Build history of the part. All positions in model axes, mm. Give positions to 0.01 mm unless a question says otherwise; leave off trailing zeros. Loops run counter-clockwise (first coordinate to the right, second up) from the corner with the lowest first, then second, coordinate; pieces in that order, holes last. Notation, with made-up numbers: M 34.25,-0.5 L 43.25,-0.5 A30 cw 43.25,21.5 Z; hole C -33.75,-17.75 d9. An arc over 180 degrees is marked long. Answer as a JSON object with one key per item and string values. Group by question number.
1. Slice it at D-D (z = 37.5). List the corners of the cut face in (x, y).
2. Slice it at A-A (x = -34). List the corners of the cut face in (y, z), then the cut area to 3 significant figures.
3. Slice it at B-B (z = -84.5). List the corners of the cut face in (x, y), then the cut area to 3 significant figures.
4. Drill centre lines: line 1 along X through (y, z) = (2.2, -101); line 2 along X through (y, z) = (2.65, 64); line 3 along X through (y, z) = (1.05, 28). Where is each one in solid material? Low to high. Write a range as [from, to].
5. Slice it at C-C (y = 1.65). Give the number of separate pieces and of enclosed holes in the cut face, then the cut area to 3 significant figures.
from build123d import *

# Parameters (mm, degrees)
SKETCH1_W            = 100
SKETCH1_H            = 210
BOSS_EXTRUDE1_DEPTH  = 3
CUT_EXTRUDE1_REACH   = 118.336
SKETCH3_R            = 1.5
SKETCH3_W            = 2
SKETCH3_H            = 100
LPATTERN1_COUNT      = 2
LPATTERN1_PITCH      = 22.5
CUT_EXTRUDE2_REACH   = 118.336
SKETCH4_W            = 20
SKETCH4_H            = 10
LPATTERN2_COUNT      = 2
LPATTERN2_PITCH      = 22.5
LPATTERN2_COUNT_DIR2 = 2
LPATTERN2_PITCH_DIR2 = 22.5
CUT_EXTRUDE3_REACH   = 118.336
SKETCH5_R            = 1.5
CUT_EXTRUDE4_REACH   = 118.336
SKETCH6_W            = 20
SKETCH6_H            = 10
LPATTERN3_COUNT      = 5
LPATTERN3_PITCH      = 15
CUT_EXTRUDE5_REACH   = 118.336
SKETCH7_R            = 1.5
CUT_EXTRUDE6_REACH   = 118.336
SKETCH8_R            = 1.5


with BuildPart() as part:
    # Sketch1 → Boss-Extrude1 (new body)
    with BuildSketch(Plane(origin=(0, 0, 0), x_dir=(1, 0, 0), z_dir=(0, 1, 0))):
        Rectangle(SKETCH1_W, SKETCH1_H)
    extrude(amount=BOSS_EXTRUDE1_DEPTH)

    # Sketch3 → Cut-Extrude1 (cut, up to next)
    with BuildSketch(Plane(origin=(0, 3, 0), x_dir=(1, 0, 0), z_dir=(0, 1, 0)), mode=Mode.PRIVATE) as cut_extrude1_sk1:
        with Locations(Location((0, -85, 0), (0, 0, 270))):
            Circle(SKETCH3_R)
    cut_extrude1_tool1 = extrude(cut_extrude1_sk1.sketch, amount=-CUT_EXTRUDE1_REACH, mode=Mode.PRIVATE) & part.part
    # Sketch3 → Cut-Extrude1 (cut, up to next)
    with BuildSketch(Plane(origin=(0, 3, 0), x_dir=(1, 0, 0), z_dir=(0, 1, 0)), mode=Mode.PRIVATE) as cut_extrude1_sk2:
        with Locations(Location((0, 35, 0), (0, 0, 270))):
            Circle(SKETCH3_R)
    cut_extrude1_tool2 = extrude(cut_extrude1_sk2.sketch, amount=-CUT_EXTRUDE1_REACH, mode=Mode.PRIVATE) & part.part
    # Sketch3 → Cut-Extrude1 (cut, up to next)
    with BuildSketch(Plane(origin=(0, 3, 0), x_dir=(1, 0, 0), z_dir=(0, 1, 0)), mode=Mode.PRIVATE) as cut_extrude1_sk3:
        with Locations((0, -25)):
            Rectangle(SKETCH3_W, SKETCH3_H)
    cut_extrude1_tool3 = extrude(cut_extrude1_sk3.sketch, amount=-CUT_EXTRUDE1_REACH, mode=Mode.PRIVATE) & part.part
    cut_extrude1_1 = cut_extrude1_tool1.solids().sort_by_distance((0, 3, 85))[0]
    add(cut_extrude1_1, mode=Mode.SUBTRACT)
    cut_extrude1_2 = cut_extrude1_tool2.solids().sort_by_distance((0, 3, -35))[0]
    add(cut_extrude1_2, mode=Mode.SUBTRACT)
    cut_extrude1_3 = cut_extrude1_tool3.solids().sort_by_distance((0, 3, 25))[0]
    add(cut_extrude1_3, mode=Mode.SUBTRACT)
    cut_extrude1 = cut_extrude1_1 + cut_extrude1_2 + cut_extrude1_3  # Cut-Extrude1 as one shape, for the pattern or mirror that repeats it

    # LPattern1: Cut-Extrude1 ×2
    with Locations(*[(i * LPATTERN1_PITCH, 0, 0) for i in range(1, LPATTERN1_COUNT)]):
        add(cut_extrude1, mode=Mode.SUBTRACT)

    # Sketch4 → Cut-Extrude2 (cut, up to next)
    with BuildSketch(Plane(origin=(0, 3, 0), x_dir=(1, 0, 0), z_dir=(0, 1, 0)), mode=Mode.PRIVATE) as cut_extrude2_sk1:
        with Locations((0, 60)):
            Rectangle(SKETCH4_W, SKETCH4_H)
    cut_extrude2_tool1 = extrude(cut_extrude2_sk1.sketch, amount=-CUT_EXTRUDE2_REACH, mode=Mode.PRIVATE) & part.part
    cut_extrude2 = cut_extrude2_tool1.solids().sort_by_distance((0, 3, -60))[0]
    add(cut_extrude2, mode=Mode.SUBTRACT)

    # LPattern2: Cut-Extrude2 2 × 2
    with Locations(*[(i * LPATTERN2_PITCH, 0, -j * LPATTERN2_PITCH_DIR2) for i in range(LPATTERN2_COUNT) for j in range(LPATTERN2_COUNT_DIR2) if (i, j) != (0, 0)]):
        add(cut_extrude2, mode=Mode.SUBTRACT)

    # Sketch5 → Cut-Extrude3 (cut, up to next)
    with BuildSketch(Plane(origin=(0, 3, 0), x_dir=(1, 0, 0), z_dir=(0, 1, 0)), mode=Mode.PRIVATE) as cut_extrude3_sk1:
        with Locations(Location((-46, 101, 0), (0, 0, 270))):
            Circle(SKETCH5_R)
    cut_extrude3_tool1 = extrude(cut_extrude3_sk1.sketch, amount=-CUT_EXTRUDE3_REACH, mode=Mode.PRIVATE) & part.part
    # Sketch5 → Cut-Extrude3 (cut, up to next)
    with BuildSketch(Plane(origin=(0, 3, 0), x_dir=(1, 0, 0), z_dir=(0, 1, 0)), mode=Mode.PRIVATE) as cut_extrude3_sk2:
        with Locations(Location((46, 101, 0), (0, 0, 270))):
            Circle(SKETCH5_R)
    cut_extrude3_tool2 = extrude(cut_extrude3_sk2.sketch, amount=-CUT_EXTRUDE3_REACH, mode=Mode.PRIVATE) & part.part
    # Sketch5 → Cut-Extrude3 (cut, up to next)
    with BuildSketch(Plane(origin=(0, 3, 0), x_dir=(1, 0, 0), z_dir=(0, 1, 0)), mode=Mode.PRIVATE) as cut_extrude3_sk3:
        with Locations(Location((46, -101, 0), (0, 0, 270))):
            Circle(SKETCH5_R)
    cut_extrude3_tool3 = extrude(cut_extrude3_sk3.sketch, amount=-CUT_EXTRUDE3_REACH, mode=Mode.PRIVATE) & part.part
    # Sketch5 → Cut-Extrude3 (cut, up to next)
    with BuildSketch(Plane(origin=(0, 3, 0), x_dir=(1, 0, 0), z_dir=(0, 1, 0)), mode=Mode.PRIVATE) as cut_extrude3_sk4:
        with Locations(Location((-46, -101, 0), (0, 0, 270))):
            Circle(SKETCH5_R)
    cut_extrude3_tool4 = extrude(cut_extrude3_sk4.sketch, amount=-CUT_EXTRUDE3_REACH, mode=Mode.PRIVATE) & part.part
    # Sketch5 → Cut-Extrude3 (cut, up to next)
    with BuildSketch(Plane(origin=(0, 3, 0), x_dir=(1, 0, 0), z_dir=(0, 1, 0)), mode=Mode.PRIVATE) as cut_extrude3_sk5:
        with Locations(Location((11.25, 0, 0), (0, 0, 270))):
            Circle(SKETCH5_R)
    cut_extrude3_tool5 = extrude(cut_extrude3_sk5.sketch, amount=-CUT_EXTRUDE3_REACH, mode=Mode.PRIVATE) & part.part
    add(cut_extrude3_tool1.solids().sort_by_distance((-46, 3, -101))[0], mode=Mode.SUBTRACT)
    add(cut_extrude3_tool2.solids().sort_by_distance((46, 3, -101))[0], mode=Mode.SUBTRACT)
    add(cut_extrude3_tool3.solids().sort_by_distance((46, 3, 101))[0], mode=Mode.SUBTRACT)
    add(cut_extrude3_tool4.solids().sort_by_distance((-46, 3, 101))[0], mode=Mode.SUBTRACT)
    add(cut_extrude3_tool5.solids().sort_by_distance((11.25, 3, 0))[0], mode=Mode.SUBTRACT)

    # Sketch6 → Cut-Extrude4 (cut, up to next)
    with BuildSketch(Plane(origin=(0, 3, 0), x_dir=(1, 0, 0), z_dir=(0, 1, 0)), mode=Mode.PRIVATE) as cut_extrude4_sk1:
        with Locations((-30, 30)):
            Rectangle(SKETCH6_W, SKETCH6_H)
    cut_extrude4_tool1 = extrude(cut_extrude4_sk1.sketch, amount=-CUT_EXTRUDE4_REACH, mode=Mode.PRIVATE) & part.part
    cut_extrude4 = cut_extrude4_tool1.solids().sort_by_distance((-30, 3, -30))[0]
    add(cut_extrude4, mode=Mode.SUBTRACT)

    # LPattern3: Cut-Extrude4 ×5
    with Locations(*[(0, 0, i * LPATTERN3_PITCH) for i in range(1, LPATTERN3_COUNT)]):
        add(cut_extrude4, mode=Mode.SUBTRACT)

    # Sketch7 → Cut-Extrude5 (cut, up to next)
    with BuildSketch(Plane(origin=(0, 3, 0), x_dir=(1, 0, 0), z_dir=(0, 1, 0)), mode=Mode.PRIVATE) as cut_extrude5_sk1:
        with Locations(Location((-46, 0, 0), (0, 0, 270))):
            Circle(SKETCH7_R)
    cut_extrude5_tool1 = extrude(cut_extrude5_sk1.sketch, amount=-CUT_EXTRUDE5_REACH, mode=Mode.PRIVATE) & part.part
    add(cut_extrude5_tool1.solids().sort_by_distance((-46, 3, 0))[0], mode=Mode.SUBTRACT)

    # Sketch8 → Cut-Extrude6 (cut, up to next)
    with BuildSketch(Plane(origin=(0, 3, 0), x_dir=(1, 0, 0), z_dir=(0, 1, 0)), mode=Mode.PRIVATE) as cut_extrude6_sk1:
        with Locations(Location((46, 0, 0), (0, 0, 270))):
            Circle(SKETCH8_R)
    cut_extrude6_tool1 = extrude(cut_extrude6_sk1.sketch, amount=-CUT_EXTRUDE6_REACH, mode=Mode.PRIVATE) & part.part
    add(cut_extrude6_tool1.solids().sort_by_distance((46, 3, 0))[0], mode=Mode.SUBTRACT)


solid = part.part
Established:
{
 "1": {"outline": "M -50,0 L -1,0 L -1,3 L -50,3 Z; M 1,0 L 21.5,0 L 21.5,3 L 1,3 Z; M 23.5,0 L 50,0 L 50,3 L 23.5,3 Z"},
 "2": {"outline": "M 0,-105 L 3,-105 L 3,-35 L 0,-35 Z; M 0,-25 L 3,-25 L 3,-20 L 0,-20 Z; M 0,-10 L 3,-10 L 3,-5 L 0,-5 Z; M 0,5 L 3,5 L 3,10 L 0,10 Z; M 0,20 L 3,20 L 3,25 L 0,25 Z; M 0,35 L 3,35 L 3,105 L 0,105 Z", "area": "480 mm^2"},
 "3": {"outline": "M -50,0 L -10,0 L -10,3 L -50,3 Z; M 10,0 L 12.5,0 L 12.5,3 L 10,3 Z; M 32.5,0 L 50,0 L 50,3 L 32.5,3 Z", "area": "180 mm^2"},
 "4": {"line 1": "x = [-50, -47.5], [-44.5, 44.5], [47.5, 50]", "line 2": "x = [-50, -1], [1, 21.5], [23.5, 50]", "line 3": "x = [-50, -40], [-20, -1], [1, 21.5], [23.5, 50]"},
 "5": {"separate pieces": "1", "enclosed holes": "22", "area": "18,700 mm^2"}
}
